Geometry check sheet. Reference: drawing and pictorial views, mm from the part's lowest x, y, z. Give positions to 0.01 mm unless a question says otherwise; leave off trailing zeros. Write each loop counter-clockwise with the first axis right and the second up, starting at its lowest first coordinate (ties: lowest second). Pieces come first, ordered by that corner, then holes. Notation, with made-up numbers: (-5.5, 57.25) -> (10.5, 57.25) arc R14 ccw to (10.5, 74.25) -> close; hole circle Ø10 at (-3, -34). An arc over 180 degrees is marked (long way). Answer as CSV lines item,"result".
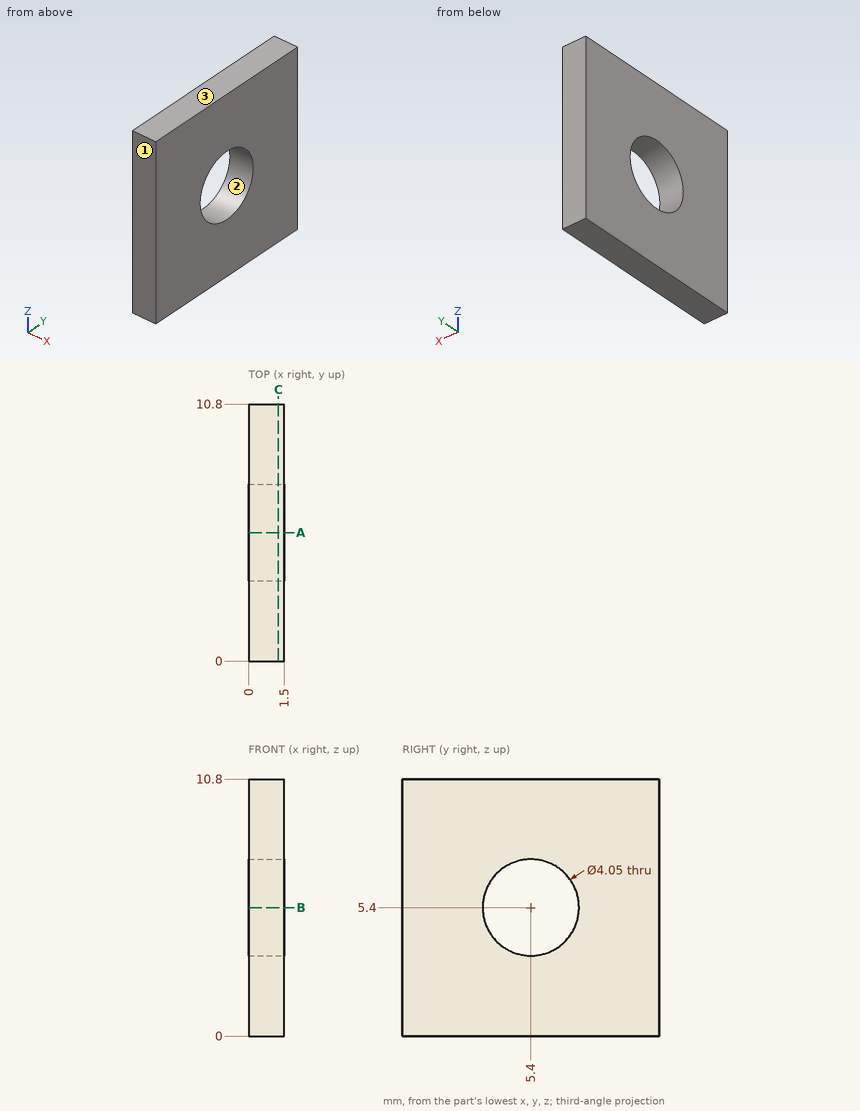
1) Section check C-C (x = 1.25). Record the boundary of the cut face in (y, z) (3 decimals).
Reported:
outline,"(0, 0) -> (10.8, 0) -> (10.8, 10.8) -> (0, 10.8) -> close; hole circle Ø4.05 at (5.4, 5.4)"
2) Scan lines: line 1 along Y through (x, z) = (0.55, 5.4) (3 decimals); line 2 along Y through (x, z) = (1.45, 4.25). Record each from-to range of solid material in increasing order.
Reported:
line 1,"0 to 3.375, 7.425 to 10.8"
line 2,"0 to 3.73, 7.07 to 10.8"
3) Section check A-A (y = 5.4). Record the boundary of the cut face in (x, z) (3 decimals).
Reported:
outline,"(0, 0) -> (1.5, 0) -> (1.5, 3.375) -> (0, 3.375) -> close; (0, 7.425) -> (1.5, 7.425) -> (1.5, 10.8) -> (0, 10.8) -> close"
4) Draft check along Y on the marked faces 1, 2 and 3. Enter one of: +Y half, -Y half, draft (parallel to the pull), parting line (faces both ways), or undercut.
Reported:
face 1,"-Y half"
face 2,"undercut"
face 3,"draft"
